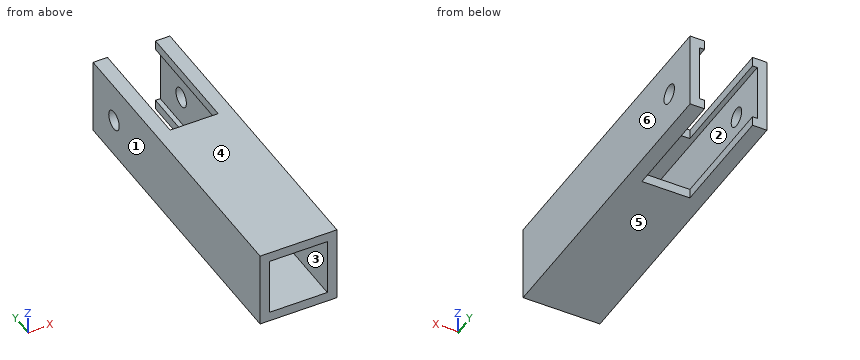
Autodesk Inventor part; units mm, degrees
ref_plane "YZ Plane" through (0, 0, 0) normal (1, 0, 0) x (0, 1, 0)
ref_plane "XZ Plane" through (0, 0, 0) normal (0, 1, 0) x (-1, 0, 0)
ref_plane "XY Plane" through (0, 0, 0) normal (0, 0, 1) x (1, 0, 0)
sketch "Sketch1" plane through (0, 0, 0) normal (0, 0, 1) x (1, 0, 0)
  line L0 (0, 0) -> (25.4, 0)
  line L1 (25.4, 0) -> (25.4, 101.6)
  line L2 (25.4, 101.6) -> (0, 101.6)
  line L3 (0, 101.6) -> (0, 0)
  dimension "d0" = 25.4
  dimension "d1" = 101.6
extrude "Extrusion1" add sketch "Sketch1" along normal blind 25.4
shell "Shell1" thickness 3.175 removed faces 2 at (16.9333, 101.6, 16.9333) at (8.4667, 0, 8.4667)
sketch "Sketch2" plane through (25.4, 0, 0) normal (1, 0, 0) x (0, 0, -1)
  line L0 (0, 0) -> (0, 101.6)
  circle A0 centre (-12.7, 88.9) radius 3.175
  line L1 (0, 0) -> (-25.4, 0)
  dimension "d8" = 6.35
  dimension "d9" = 12.7
  dimension "d13" = 88.9
extrude "Extrusion2" cut sketch "Sketch2" against normal through all
sketch "Sketch3" plane through (0, 0, 0) normal (0, 0, -1) x (-1, 0, 0)
  line L0 (0, 101.6) -> (0, 0)
  line L1 (-25.4, 101.6) -> (0, 101.6)
  line L2 (-25.4, 0) -> (-25.4, 101.6)
  line L3 (-20.6375, 101.6) -> (-4.7625, 101.6)
  line L4 (-4.7625, 101.6) -> (-4.7625, 63.5)
  line L5 (-4.7625, 63.5) -> (-20.6375, 63.5)
  line L6 (-20.6375, 63.5) -> (-20.6375, 101.6)
  dimension "d14" = 38.1
  dimension "d15" = 4.7625
  dimension "d16" = 4.7625
extrude "Extrusion3" cut sketch "Sketch3" against normal blind 25.4
properties part number "PivotLeverBar" material "Aluminum-6061"
Input: part model. Units: mm. Frame: model coordinates. Face numbers are marked on the shaded views. A direction names the side the tool comes from. Give positions to 0.01 mm unless a question says otherwise; leave off trailing zeros. Loops run counter-clockwise (first coordinate to the right, second up) from the corner with the lowest first, then second, coordinate; pieces in that order, holes last. Notation, with made-up numbers: M -32.75,27.25 L -4.75,27.25 A22 cw -4.75,36.25 Z; hole C 84,7.5 d3. An arc over 180 degrees is marked long. Use one line per item in the form item = value.
1. First-contact query: pin 1 (8 mm diameter, centred on x = 9, y = 70, fed in from +Z); pin 2 (2.5 mm diameter, centred on x = 14, z = 2, fed in from +Y). Flat tips, straight axial feed; report the tip coordinate or a pass-through.
Numbers:
pin_1 = through
pin_2 = 63.5
2. Reachability of the marked faces 1 and 2 from +Z, -Z, +X, -X, +Y, -Y: full face, straight path, thin tool, end or side. Return the list, or none.
Numbers:
face_1 = +Z, -Z, -X, +Y, -Y
face_2 = +Y, -Y
3. Section query C-C, the plane z = 12.7. Return the cut outline in (x, y) (3 decimals), and give its area (3 significant figures).
Numbers:
outline = M 0,0 L 3.175,0 L 3.175,85.725 L 0,85.725 Z; M 0,92.075 L 3.175,92.075 L 3.175,101.6 L 0,101.6 Z; M 22.225,0 L 25.4,0 L 25.4,85.725 L 22.225,85.725 Z; M 22.225,92.075 L 25.4,92.075 L 25.4,101.6 L 22.225,101.6 Z
area = 605 mm²
4. Line query: L1, parallel to X at y = 12, z = 8.25 (3 decimals); L2, parallel to Y at x = 0.85, z = 12.7 (3 decimals). Output: solid intervals per line, ascending.
Numbers:
L1 = 0 to 3.175, 22.225 to 25.4
L2 = 0 to 85.725, 92.075 to 101.6
5. Pull-direction query (Z, two-part tool) for the marked faces 3, 4, 5 and 6; classes: released by +Z, released by -Z, zero draft, split by the parting line, or undercut.
Numbers:
face_3 = undercut
face_4 = released by +Z
face_5 = released by -Z
face_6 = zero draft
6. Section query B-B, the plane z = 5.5. Return the cut outline in (x, y) (3 decimals).
Numbers:
outline = M 0,0 L 3.175,0 L 3.175,101.6 L 0,101.6 Z; M 22.225,0 L 25.4,0 L 25.4,101.6 L 22.225,101.6 Z
7. Section query A-A, the plane y = 88.9. Return the cut outline in (x, z) (1 decimal), and give its area (3 significant figures).
Numbers:
outline = M 0,0 L 4.8,0 L 4.8,3.2 L 3.2,3.2 L 3.2,9.5 L 0,9.5 Z; M 0,15.9 L 3.2,15.9 L 3.2,22.2 L 4.8,22.2 L 4.8,25.4 L 0,25.4 Z; M 20.6,0 L 25.4,0 L 25.4,9.5 L 22.2,9.5 L 22.2,3.2 L 20.6,3.2 Z; M 20.6,22.2 L 22.2,22.2 L 22.2,15.9 L 25.4,15.9 L 25.4,25.4 L 20.6,25.4 Z
area = 141 mm²
8. Section query D-D, the plane x = 11.25. Return the cut outline in (y, z) (3 decimals), and give its area (3 significant figures).
Numbers:
outline = M 0,0 L 63.5,0 L 63.5,3.175 L 0,3.175 Z; M 0,22.225 L 63.5,22.225 L 63.5,25.4 L 0,25.4 Z
area = 403 mm²
